from build123d import *

# Parameters (mm, degrees)
ESQUISSE1_W               = 40.2629848
ESQUISSE1_H               = 26.817935246
BOSS_EXTRU_1_DEPTH        = 65
COQUE1_T                  = -1.5
COQUE1_THICKNESS_2_FACE_W = 63.5
COQUE1_THICKNESS_2_FACE_H = 25.317935246
COQUE1_THICKNESS_2_DEPTH  = 3.45
COQUE1_THICKNESS_3_FACE_W = 25.317935246
COQUE1_THICKNESS_3_FACE_H = 63.5
COQUE1_THICKNESS_3_DEPTH  = 3.45
COQUE1_THICKNESS_4_FACE_W = 63.5
COQUE1_THICKNESS_4_FACE_H = 30.3629848
COQUE1_THICKNESS_4_DEPTH  = 8.5
COQUE1_THICKNESS_5_FACE_W = 30.3629848
COQUE1_THICKNESS_5_FACE_H = 16.817935246
COQUE1_THICKNESS_5_DEPTH  = 3.5
ESQUISSE4_W               = 40.2629848
ESQUISSE4_H               = 65
BOSS_EXTRU_2_DEPTH        = 2
ESQUISSE5_R               = 4.065
ENL_V_MAT_EXTRU_3_DEPTH   = 82.026598076
CONG_2_R                  = 10
CONG_3_R                  = 10
ESQUISSE6_W               = 16
ESQUISSE6_H               = 16.817935246
ENL_V_MAT_EXTRU_4_DEPTH   = 78.073403946


with BuildPart() as part:
    # Esquisse1 → Boss.-Extru.1 (new body)
    with BuildSketch(Plane.XY):
        with Locations((20.1314924, 13.408967623)):
            Rectangle(ESQUISSE1_W, ESQUISSE1_H)
    extrude(amount=BOSS_EXTRU_1_DEPTH)

    # Coque1
    coque1_openings = [part.faces().sort_by_distance(p)[0] for p in [
        (20.1314924, 13.408967623, 65),
        (20.1314924, 26.817935246, 32.5),
    ]]
    offset(amount=COQUE1_T, openings=coque1_openings, kind=Kind.INTERSECTION)

    # Coque1 thickness 2 face (on inner face of the shell) → Coque1 thickness 2 (add)
    with BuildSketch(Plane(origin=(1.5, 14.158967623, 33.25), x_dir=(0, 0, -1), z_dir=(-1, 0, 0))):
        Rectangle(COQUE1_THICKNESS_2_FACE_W, COQUE1_THICKNESS_2_FACE_H)
    extrude(amount=-COQUE1_THICKNESS_2_DEPTH)

    # Coque1 thickness 3 face (on inner face of the shell) → Coque1 thickness 3 (add)
    with BuildSketch(Plane(origin=(38.7629848, 14.158967623, 33.25), x_dir=(0, 1, 0), z_dir=(1, 0, 0))):
        Rectangle(COQUE1_THICKNESS_3_FACE_W, COQUE1_THICKNESS_3_FACE_H)
    extrude(amount=-COQUE1_THICKNESS_3_DEPTH)

    # Coque1 thickness 4 face (on inner face of the shell) → Coque1 thickness 4 (add)
    with BuildSketch(Plane(origin=(20.1314924, 1.5, 33.25), x_dir=(0, 0, -1), z_dir=(0, -1, 0))):
        Rectangle(COQUE1_THICKNESS_4_FACE_W, COQUE1_THICKNESS_4_FACE_H)
    extrude(amount=-COQUE1_THICKNESS_4_DEPTH)

    # Coque1 thickness 5 face (on inner face of the shell) → Coque1 thickness 5 (add)
    with BuildSketch(Plane(origin=(20.1314924, 18.408967623, 1.5), x_dir=(-1, 0, 0), z_dir=(0, 0, -1))):
        Rectangle(COQUE1_THICKNESS_5_FACE_W, COQUE1_THICKNESS_5_FACE_H)
    extrude(amount=-COQUE1_THICKNESS_5_DEPTH)

    # Esquisse4 → Boss.-Extru.2 (add)
    with BuildSketch(Plane.XZ):
        with Locations((20.1314924, 32.5)):
            Rectangle(ESQUISSE4_W, ESQUISSE4_H)
    extrude(amount=BOSS_EXTRU_2_DEPTH)

    # Esquisse5 → Enlèv. mat.-Extru.3 (cut, through all)
    with BuildSketch(Plane(origin=(40.2629848, 0, 0), x_dir=(0, 0, -1), z_dir=(1, 0, 0))):
        with Locations((-15, 5)):
            Circle(ESQUISSE5_R)
        with Locations((-45, 5)):
            Circle(ESQUISSE5_R)
    extrude(amount=-ENL_V_MAT_EXTRU_3_DEPTH, mode=Mode.SUBTRACT)

    # Congé2
    cong_2_edges = [part.edges().sort_by_distance(p)[0] for p in [
        (20.1314924, -2, 0),
    ]]
    fillet(cong_2_edges, radius=CONG_2_R)

    # Congé3
    cong_3_edges = [part.edges().sort_by_distance(p)[0] for p in [
        (20.1314924, -2, 65),
    ]]
    fillet(cong_3_edges, radius=CONG_3_R)

    # Esquisse6 → Enlèv. mat.-Extru.4 (cut, through all)
    with BuildSketch(Plane.XY.offset(5)):
        with Locations((27.3129848, 18.408967623)):
            Rectangle(ESQUISSE6_W, ESQUISSE6_H)
    extrude(amount=-ENL_V_MAT_EXTRU_4_DEPTH, mode=Mode.SUBTRACT)


solid = part.part
The listing builds one solid part. Answer for the finished solid, in the listing's coordinates (mm). A direction names the side the tool comes from. Give positions to 0.01 mm unless a question says otherwise; leave off trailing zeros. Write each loop counter-clockwise with the first axis right and the second up, starting at its lowest first coordinate (ties: lowest second). Pieces come first, ordered by that corner, then holes. Notation, with made-up numbers: (78.5, -5.5) -> (134.5, -5.5) arc R21 ccw to (134.5, 21.5) -> close; hole circle Ø8 at (84, 5). An arc over 180 degrees is marked (long way). Use a Markdown table: item, result.
(1) Flat-ended cylindrical pins translate along their axes: P1, Ø8, axis at x = 22.5, z = 38.5, coming from the +Y side; P2, Ø4.5, axis at x = 14, y = 20.5, coming from the +Z side. Find the tip coordinate at first contact, or state that the pin passes through.
Return value:
| item | result |
|---|---|
| P1 | y = 10 |
| P2 | z = 5 |
(2) Determine the mould class of faces 1 (the flat face through (38, 26.818, 32)), 2 (the cylindrical face through (20.413, 6.221, 11.123)), 3 (the flat face through (19.313, 18, 3)), 4 (the cylindrical face through (20.41, 5.18, 49.06)) for opening direction Y: released by +Y, released by -Y, zero draft, split by the parting line, or undercut.
Return value:
| item | result |
|---|---|
| face 1 | released by +Y |
| face 2 | undercut |
| face 3 | zero draft |
| face 4 | undercut |
(3) Section A-A, the plane x = 24 is taken. Determine the outline of the cut face in (y, z) (3 decimals).
Return value:
| item | result |
|---|---|
| outline | (-2, 10) arc R10 ccw to (8, 0) -> (10, 0) -> (10, 65) -> (8, 65) arc R10 ccw to (-2, 55) -> close; hole circle Ø8.13 at (5, 15); hole circle Ø8.13 at (5, 45) |
(4) Section C-C, the plane z = 45 is taken. Determine the outline of the cut face in (x, y) (3 decimals).
Return value:
| item | result |
|---|---|
| outline | (0, -2) -> (40.263, -2) -> (40.263, 0.935) -> (0, 0.935) -> close; (0, 9.065) -> (40.263, 9.065) -> (40.263, 26.818) -> (35.313, 26.818) -> (35.313, 10) -> (4.95, 10) -> (4.95, 26.818) -> (0, 26.818) -> close |
(5) Find the intervals of material crossed by probe 1 along Y at (x, z) = (24, 45) (3 decimals); probe 2 along X at (y, z) = (23, 42), in increasing order. Write a range as from..to.
Return value:
| item | result |
|---|---|
| probe 1 | -2..0.935, 9.065..10 |
| probe 2 | 0..4.95, 35.31..40.26 |
(6) For faces 5 (the flat face through (12, 19, 5)), 6 (the flat face through (20, -2, 33)), 7 (the flat face through (35.313, 18, 33)), determine the directions among +Z, -Z, +X, -X, +Y, -Y from which every point of the face is accessible in a straight line to the end or side of a thin tool.
Return value:
| item | result |
|---|---|
| face 5 | +Z, +Y |
| face 6 | +Z, -Z, +X, -X, -Y |
| face 7 | +Z, -Z, +Y |
(7) Section D-D, the plane z = 24 is taken. Determine the outline of the cut face in (x, y).
Return value:
| item | result |
|---|---|
| outline | (0, -2) -> (40.26, -2) -> (40.26, 26.82) -> (35.31, 26.82) -> (35.31, 10) -> (4.95, 10) -> (4.95, 26.82) -> (0, 26.82) -> close |
(8) Section B-B, the plane y = 12 is taken. Determine the outline of the cut face in (x, z), then the cut area to 3 significant figures.
Return value:
| item | result |
|---|---|
| outline | (0, 0) -> (19.31, 0) -> (19.31, 5) -> (4.95, 5) -> (4.95, 65) -> (0, 65) -> close; (35.31, 0) -> (40.26, 0) -> (40.26, 65) -> (35.31, 65) -> close |
| area | 715 mm2 |
